Source: CAD feature listing. Evaluate the final solid. Frame: model axes, mm. Round coordinates to 2 decimals unless told otherwise and drop trailing zeros. Loops run counter-clockwise (first coordinate to the right, second up) from the corner with the lowest first, then second, coordinate; pieces in that order, holes last. Notation, with made-up numbers: (16.5, 23) -> (46.5, 23) arc R29 cw to (46.5, 45) -> close; hole circle Ø8 at (83.25, -22.75). An arc over 180 degrees is marked (long way). Put each result on its own line as item: value. Start each with the question number.
1. Cut plane A-A (y = -43). Return the cut outline in (x, z), then the cut area to 3 significant figures.
2. Cut plane D-D (z = 1.5). State how many separate pieces and enclosed holes the cut face has, then the cut area to 3 significant figures.
3. Material intervals for L1, parallel to Y at x = -9, z = 1.15; L2, parallel to Y at x = -10, z = 2.65; L3, parallel to X at y = -49.5, z = 0.2, sorted ascending.
4. Contact query for flat-ended pins moving along their axis: pin 1 (1.5 mm diameter, centred on x = -30, z = 1, fed in from -Y); pin 2 (0.9 mm diameter, centred on x = -29, z = 2, fed in from +Y); pin 3 (0.9 mm diameter, centred on y = -70.5, z = 2, fed in from +X). Output: stop coordinate, or through.
5. Cut plane B-B (x = -21.5). Return the cut outline in (y, z), then the cut area to 3 significant figures.
6. Cut plane C-C (x = -10.5). Return the cut outline in (y, z).
```python
from build123d import *

# Parameters (mm, degrees)
ESQUISSE1_R        = 8.5
ESQUISSE1_W        = 4
ESQUISSE1_H        = 10
BOSS_EXTRU_1_DEPTH = 3


with BuildPart() as part:
    # Esquisse1 → Boss.-Extru.1 (new body)
    with BuildSketch(Plane.XY):
        Polygon((2.029381216, -75.048859935), (-27.970618784, -75.048859935), (-27.970618784, -65.048859935), (-30.970618784, -65.048859935), (-30.970618784, -55.048859935), (-27.970618784, -55.048859935), (-27.970618784, -40.048859935), (-30.970618784, -40.048859935), (-30.970618784, -30.048859935), (-27.970618784, -30.048859935), (-27.970618784, -15.048859935), (-30.970618784, -15.048859935), (-30.970618784, -5.048859935), (-27.970618784, -5.048859935), (-27.970618784, 9.951140065), (-30.970618784, 9.951140065), (-30.970618784, 19.951140065), (-27.970618784, 19.951140065), (-27.970618784, 34.951140065), (-30.970618784, 34.951140065), (-30.970618784, 44.951140065), (-27.970618784, 44.951140065), (-27.970618784, 54.951140065), (-17.970618784, 54.951140065), (-17.970618784, 51.951140065), (-7.970618784, 51.951140065), (-7.970618784, 54.951140065), (2.029381216, 54.951140065), (2.029381216, 44.951140065), (5.029381216, 44.951140065), (5.029381216, 34.951140065), (2.029381216, 34.951140065), (2.029381216, 19.951140065), (5.029381216, 19.951140065), (5.029381216, 9.951140065), (2.029381216, 9.951140065), (2.029381216, -5.048859935), (5.029381216, -5.048859935), (5.029381216, -15.048859935), (2.029381216, -15.048859935), (2.029381216, -30.048859935), (5.029381216, -30.048859935), (5.029381216, -40.048859935), (2.029381216, -40.048859935), (2.029381216, -55.048859935), (5.029381216, -55.048859935), (5.029381216, -65.048859935), (2.029381216, -65.048859935), align=None)
        with Locations((-8.970618784, 39.768013852)):
            Circle(ESQUISSE1_R, mode=Mode.SUBTRACT)
        with Locations((-8.970618784, 13.468013852)):
            Circle(ESQUISSE1_R, mode=Mode.SUBTRACT)
        with Locations((-20.834297512, -45.048859935)):
            Rectangle(ESQUISSE1_W, ESQUISSE1_H, mode=Mode.SUBTRACT)
    extrude(amount=BOSS_EXTRU_1_DEPTH)


solid = part.part
```
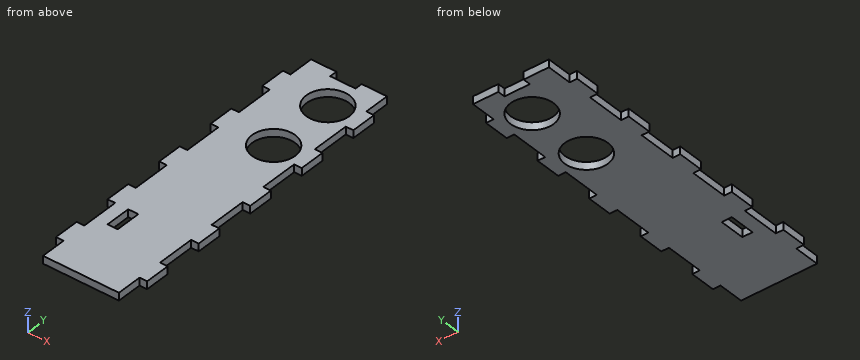
Solution:
1. outline: (-27.97, 0) -> (-22.83, 0) -> (-22.83, 3) -> (-27.97, 3) -> close; (-18.83, 0) -> (2.03, 0) -> (2.03, 3) -> (-18.83, 3) -> close
1. area: 78.0 mm^2
2. separate pieces: 1
2. enclosed holes: 3
2. area: 3,680 mm^2
3. L1: y = -75.05 to 4.97, 21.97 to 31.27, 48.27 to 51.95
3. L2: y = -75.05 to 5.03, 21.91 to 31.33, 48.21 to 51.95
3. L3: x = -27.97 to -22.83, -18.83 to 2.03
4. pin 1: stops at y = -65.05
4. pin 2: stops at y = 44.95
4. pin 3: stops at x = 2.03
5. outline: (-75.05, 0) -> (-50.05, 0) -> (-50.05, 3) -> (-75.05, 3) -> close; (-40.05, 0) -> (54.95, 0) -> (54.95, 3) -> (-40.05, 3) -> close
5. area: 360 mm^2
6. outline: (-75.05, 0) -> (5.11, 0) -> (5.11, 3) -> (-75.05, 3) -> close; (21.83, 0) -> (31.41, 0) -> (31.41, 3) -> (21.83, 3) -> close; (48.13, 0) -> (51.95, 0) -> (51.95, 3) -> (48.13, 3) -> close
